Verification items for the finished model (mm, model axes). A direction names the side the tool comes from. Coordinates: 2 decimals unless noted, no trailing zeros. Order: outer loops, then holes, each group sorted by start corner. A loop starts at its lowest first (then second) coordinate and runs counter-clockwise, first axis right, second up. Notation, with made-up numbers: M -10.5,26.25 L -3.5,26.25 A10 ccw -3.5,32.25 Z; hole C -36,-34.75 d11. An arc over 180 degrees is marked long. Write item = value, one per line.
```python
from build123d import *

# Parameters (mm, degrees)
BOSS_EXTRUDE1_DEPTH = 32
CUT_EXTRUDE1_DEPTH  = 28
SKETCH3_R           = 5
BOSS_EXTRUDE2_DEPTH = 23
SKETCH4_R           = 1.9
BOSS_EXTRUDE3_DEPTH = 10
BOSS_EXTRUDE4_DEPTH = 9
BOSS_EXTRUDE6_DEPTH = 28
SKETCH7_W           = 45
SKETCH7_H           = 22
CUT_EXTRUDE2_DEPTH  = 5
CHAMFER1_SIZE       = 5
SKETCH8_R           = 2.5
SKETCH8_W           = 6
SKETCH8_H           = 6
CUT_EXTRUDE3_DEPTH  = 5
SKETCH10_R          = 1.17
SKETCH10_R_2        = 1.043
BOSS_EXTRUDE8_DEPTH = 8
SKETCH11_W          = 12
SKETCH11_H          = 10
CUT_EXTRUDE4_DEPTH  = 8
SKETCH12_W          = 10
SKETCH12_H          = 10
CUT_EXTRUDE5_DEPTH  = 8
SKETCH16_W          = 22.284271248
SKETCH16_H          = 29
CUT_EXTRUDE6_DEPTH  = 0.5
SKETCH17_W          = 54
SKETCH17_H          = 29
CUT_EXTRUDE7_DEPTH  = 0.5
SKETCH18_W          = 22.284271248
SKETCH18_H          = 29
CUT_EXTRUDE8_DEPTH  = 0.5
SKETCH19_W          = 54
SKETCH19_H          = 29
CUT_EXTRUDE9_DEPTH  = 0.5


with BuildPart() as part:
    # Sketch1 → Boss-Extrude1 (new body)
    with BuildSketch(Plane(origin=(0, 0, 0), x_dir=(1, 0, 0), z_dir=(0, 1, 0))):
        Polygon((30, 50), (-30, 50), (-50, 30), (-50, -30), (-30, -50), (30, -50), (50, -30), (50, 30), align=None)
    extrude(amount=BOSS_EXTRUDE1_DEPTH)

    # Sketch2 → Cut-Extrude1 (cut)
    with BuildSketch(Plane(origin=(0, 32, 0), x_dir=(1, 0, 0), z_dir=(0, 1, 0))):
        Polygon((-28.757359313, -47), (28.757359313, -47), (47, -28.757359313), (47, 28.757359313), (28.757359313, 47), (-28.757359313, 47), (-47, 28.757359313), (-47, -28.757359313), align=None)
    extrude(amount=-CUT_EXTRUDE1_DEPTH, mode=Mode.SUBTRACT)

    # Sketch3 → Boss-Extrude2 (add)
    with BuildSketch(Plane(origin=(0, 4, 0), x_dir=(1, 0, 0), z_dir=(0, 1, 0))):
        with Locations(Location((0, 0, 0), (0, 0, 270))):
            Circle(SKETCH3_R)
    extrude(amount=BOSS_EXTRUDE2_DEPTH)

    # Sketch4 → Boss-Extrude3 (add)
    with BuildSketch(Plane(origin=(0, 27, 0), x_dir=(1, 0, 0), z_dir=(0, 1, 0))):
        with Locations(Location((0, 0, 0), (0, 0, 270))):
            Circle(SKETCH4_R)
    extrude(amount=BOSS_EXTRUDE3_DEPTH)

    # Sketch5 → Boss-Extrude4 (add)
    with BuildSketch(Plane(origin=(0, 4, 0), x_dir=(1, 0, 0), z_dir=(0, 1, 0))):
        Polygon((-16.970562748, 8.838834765), (-31.112698372, 22.980970389), (-22.980970389, 31.112698372), (-8.838834765, 16.970562748), (-7.424621202, 18.384776311), (-22.980970389, 33.941125497), (-33.941125497, 22.980970389), (-18.384776311, 7.424621202), align=None)
    extrude(amount=BOSS_EXTRUDE4_DEPTH)

    # Sketch6 → Boss-Extrude6 (add)
    with BuildSketch(Plane(origin=(0, 4, 0), x_dir=(1, 0, 0), z_dir=(0, 1, 0))):
        Polygon((42, -33.757359313), (47, -28.757359313), (47, 28.757359313), (42, 33.757359313), align=None)
    extrude(amount=BOSS_EXTRUDE6_DEPTH)

    # Sketch7 → Cut-Extrude2 (cut)
    with BuildSketch(Plane(origin=(50, 0, 0), x_dir=(0, 0, -1), z_dir=(1, 0, 0))):
        with Locations((0, 16)):
            Rectangle(SKETCH7_W, SKETCH7_H)
    extrude(amount=-CUT_EXTRUDE2_DEPTH, mode=Mode.SUBTRACT)

    # Chamfer1
    chamfer1_edges = [part.edges().sort_by_distance(p)[0] for p in [
        (50, 16, 22.5),
        (50, 27, 0),
        (50, 16, -22.5),
        (50, 5, 0),
    ]]
    chamfer(chamfer1_edges, length=CHAMFER1_SIZE - 0.0001)  # a hair under: the kernel refuses the full size

    # Sketch8 → Cut-Extrude3 (cut)
    with BuildSketch(Plane(origin=(45, 0, 0), x_dir=(0, 0, -1), z_dir=(1, 0, 0))):
        with Locations((-15, 21)):
            Circle(SKETCH8_R)
        with Locations((-5, 21)):
            Circle(SKETCH8_R)
        with Locations((5, 21)):
            Circle(SKETCH8_R)
        with Locations((15, 21)):
            Circle(SKETCH8_R)
        with Locations((-15, 11)):
            Rectangle(SKETCH8_W, SKETCH8_H)
        with Locations((-5, 11)):
            Rectangle(SKETCH8_W, SKETCH8_H)
        with Locations((5, 11)):
            Rectangle(SKETCH8_W, SKETCH8_H)
        with Locations((15, 11)):
            Rectangle(SKETCH8_W, SKETCH8_H)
    extrude(amount=-CUT_EXTRUDE3_DEPTH, mode=Mode.SUBTRACT)

    # Sketch10 → Boss-Extrude8 (add)
    with BuildSketch(Plane(origin=(0, 4, 0), x_dir=(1, 0, 0), z_dir=(0, 1, 0))):
        with Locations(Location((-44.46, -14.06, 0), (0, 0, 270))):
            Circle(SKETCH10_R)
        with Locations(Location((-44.46, 1.18, 0), (0, 0, 270))):
            Circle(SKETCH10_R)
        with Locations(Location((-16.52, 1.18, 0), (0, 0, 270))):
            Circle(SKETCH10_R)
        with Locations(Location((-16.52, -14.06, 0), (0, 0, 270))):
            Circle(SKETCH10_R)
        with Locations(Location((-23.738640687, -44.46, 0), (0, 0, 270))):
            Circle(SKETCH10_R_2)
        with Locations(Location((-23.738640687, -24.14, 0), (0, 0, 270))):
            Circle(SKETCH10_R_2)
        Polygon((28.757359313, -3.8), (28.757359313, -47), (31.757359313, -44), (31.757359313, -0.8), (29.355483266, -0.8), (25.717542729, -0.8), (7.757359313, -0.8), (7.757359313, -21.6), (7.757359313, -47), (10.757359313, -47), (10.757359313, -3.8), align=None)
        with BuildLine():
            Line((25.717542729, -0.8), (29.355483266, -0.8))
            Line((29.355483266, -0.8), (-4.475041798, 21.465344683))
            ThreePointArc((-4.475041798, 21.465344683), (-7.758981907, 37.393801525), (8.169474935, 40.677741633))
            Line((8.169474935, 40.677741633), (42, 18.41239695))
            Line((42, 18.41239695), (42, 20.806684353))
            Line((42, 20.806684353), (9.26899813, 42.348384846))
            ThreePointArc((9.26899813, 42.348384846), (5.919661645, 43.942642222), (2.262859211, 44.565143167))
            ThreePointArc((2.262859211, 44.565143167), (-0.878722589, 44.293466456), (-3.871580373, 43.300417249))
            ThreePointArc((-3.871580373, 43.300417249), (-6.983976281, 41.282323386), (-9.429625069, 38.493324796))
            ThreePointArc((-9.429625069, 38.493324796), (-11.023882481, 35.143988278), (-11.64638344, 31.4871858))
            ThreePointArc((-11.64638344, 31.4871858), (-11.37470673, 28.345604), (-10.381657523, 25.352746216))
            ThreePointArc((-10.381657523, 25.352746216), (-8.363563629, 22.240350274), (-5.574564992, 19.79470147))
            Line((-5.574564992, 19.79470147), (25.717542729, -0.8))
        make_face()
    extrude(amount=BOSS_EXTRUDE8_DEPTH)

    # Sketch11 → Cut-Extrude4 (cut)
    with BuildSketch(Plane(origin=(0, 0, 47), x_dir=(-1, 0, 0), z_dir=(0, 0, -1))):
        with Locations((-19.757359313, 9)):
            Rectangle(SKETCH11_W, SKETCH11_H)
    extrude(amount=-CUT_EXTRUDE4_DEPTH, mode=Mode.SUBTRACT)

    # Sketch12 → Cut-Extrude5 (cut)
    with BuildSketch(Plane(origin=(0, 4, 0), x_dir=(1, 0, 0), z_dir=(0, 1, 0))):
        with Locations((19.757359313, -20)):
            Rectangle(SKETCH12_W, SKETCH12_H)
    extrude(amount=-CUT_EXTRUDE5_DEPTH, mode=Mode.SUBTRACT)

    # Sketch16 → Cut-Extrude6 (cut)
    with BuildSketch(Plane(origin=(-40, 0, -40), x_dir=(-0.7071067811865475, 0, 0.7071067811865477), z_dir=(-0.7071067811865477, 0, -0.7071067811865475))):
        with Locations((0, 17.5)):
            Rectangle(SKETCH16_W, SKETCH16_H)
    cut_extrude6 = extrude(amount=-CUT_EXTRUDE6_DEPTH, mode=Mode.SUBTRACT)

    # Sketch17 → Cut-Extrude7 (cut)
    with BuildSketch(Plane(origin=(0, 0, -50), x_dir=(-1, 0, 0), z_dir=(0, 0, -1))):
        with Locations((0, 17.5)):
            Rectangle(SKETCH17_W, SKETCH17_H)
    cut_extrude7 = extrude(amount=-CUT_EXTRUDE7_DEPTH, mode=Mode.SUBTRACT)

    # Sketch18 → Cut-Extrude8 (cut)
    with BuildSketch(Plane(origin=(40, 0, -40), x_dir=(-0.7071067811865475, 0, -0.7071067811865477), z_dir=(0.7071067811865477, 0, -0.7071067811865475))):
        with Locations((0, 17.5)):
            Rectangle(SKETCH18_W, SKETCH18_H)
    cut_extrude8 = extrude(amount=-CUT_EXTRUDE8_DEPTH, mode=Mode.SUBTRACT)

    # Mirror1: Cut-Extrude6, Cut-Extrude7, Cut-Extrude8 across plane
    add(cut_extrude6.mirror(Plane.XY), mode=Mode.SUBTRACT)
    add(cut_extrude7.mirror(Plane.XY), mode=Mode.SUBTRACT)
    add(cut_extrude8.mirror(Plane.XY), mode=Mode.SUBTRACT)

    # Sketch19 → Cut-Extrude9 (cut)
    with BuildSketch(Plane.ZY.offset(50)):
        with Locations((0, 17.5)):
            Rectangle(SKETCH19_W, SKETCH19_H)
    extrude(amount=-CUT_EXTRUDE9_DEPTH, mode=Mode.SUBTRACT)


solid = part.part
```
Item 1: Scan lines: L1, parallel to Y at x = 44.4, z = -5; L2, parallel to X at y = 29, z = -15; L3, parallel to Z at x = -24, y = 7.5. Record each from-to range of solid material in increasing order. Write a range as from..to.
Report:
L1 = 0..8, 14..18.5, 23.5..32
L2 = -49.5..-47, 42..47
L3 = -49.5..-47, -32.92..-30.09, -15.87..-13.04, 23.13..25.15, 43.45..45.47, 47..49.5
Item 2: Sectioned sample at A-A, the plane z = -15. Give the number of separate pieces and of enclosed holes in the cut face, then the cut area to 3 significant figures.
Report:
separate_pieces = 3
enclosed_holes = 0
area = 580 mm^2
Item 3: Sectioned sample at C-C, the plane x = -44.46. Enter the section's corners in (y, z).
Report:
outline = M 0,-35.54 L 3,-35.54 L 3,-34.83 L 32,-34.83 L 32,-31.3 L 4,-31.3 L 4,-2.35 L 12,-2.35 L 12,-0.01 L 4,-0.01 L 4,12.89 L 12,12.89 L 12,15.23 L 4,15.23 L 4,31.3 L 32,31.3 L 32,34.83 L 3,34.83 L 3,35.54 L 0,35.54 Z
Item 4: Gauge pin test, flat ends, axial feed: pin 1 (4 mm diameter, centred on x = 18.5, y = 9.5, fed in from +Z); pin 2 (8 mm diameter, centred on x = -12.5, z = -18.5, fed in from +Y); pin 3 (5 mm diameter, centred on x = 36, z = 39.5, fed in from +Y). Record the tip position at first contact, or that the pin passes through.
Report:
pin_1 = 3.8
pin_2 = 13
pin_3 = 32
Item 5: Release check for a two-part mould opening along Z. For faces 4 (the flat face through (50, 16, -29)), 5 (the cylindrical face through (43.52, 22.69, 16.84)), 6 (the flat face through (39, 2, -41)) record: pulls with the +Z half, pulls with the -Z half, needs draft (parallel to the pull), parting line crosses it, or undercut.
Report:
face_4 = needs draft
face_5 = undercut
face_6 = pulls with the -Z half
Item 6: Tool access check on faces 1 (the flat face through (20, 2, 25)), 2 (the flat face through (7.757, 8, 24)), 3 (the flat face through (44, 8, -15)). Record the directions out of +Z, -Z, +X, -X, +Y, -Y that give a thin tool (end or side, any length) a straight path to the whole face; none if there is none.
Report:
face_1 = +Y, -Y
face_2 = +Y
face_3 = +X
